Input: part model. Units: mm. Frame: model coordinates. A direction names the side the tool comes from. Coordinates: 2 decimals unless noted, no trailing zeros. Order: outer loops, then holes, each group sorted by start corner. A loop starts at its lowest first (then second) coordinate and runs counter-clockwise, first axis right, second up. Notation, with made-up numbers: M 57,-13 L 64,-13 A27 cw 64,8 Z; hole C 52.25,-15.5 d9. An arc over 180 degrees is marked long. Answer in a Markdown table with one row per item.
from build123d import *

# Parameters (mm, degrees)
F1_DEPTH = 9.271
F2_R     = 6.731
F3_DEPTH = 6.35


with BuildPart() as f1:
    # F0 (on Top) → F1 (new body)
    with BuildSketch(Plane.XY):
        with BuildLine():
            Line((16.51, 19.05), (-16.51, 19.05))
            ThreePointArc((-16.51, 19.05), (-18.306051, 18.306051), (-19.05, 16.51))
            Line((-19.05, 16.51), (-19.05, -16.51))
            ThreePointArc((-19.05, -16.51), (-18.306051, -18.306051), (-16.51, -19.05))
            Line((-16.51, -19.05), (16.51, -19.05))
            ThreePointArc((16.51, -19.05), (18.306051, -18.306051), (19.05, -16.51))
            Line((19.05, -16.51), (19.05, 16.51))
            ThreePointArc((19.05, 16.51), (18.306051, 18.306051), (16.51, 19.05))
        make_face()
    extrude(amount=F1_DEPTH)

    # F2 (on face) → F3 (cut)
    with BuildSketch(Plane.XY.offset(9.271)):
        Circle(F2_R)
    extrude(amount=-F3_DEPTH, mode=Mode.SUBTRACT)


solid = f1.part
1) Contact query for flat-ended pins moving along their axis: pin 1 (3 mm diameter, centred on x = -5, y = 15, fed in from -Z); pin 2 (6.5 mm diameter, centred on x = -1, y = 2, fed in from +Z). Output: stop coordinate, or through.
Resolved:
| item | result |
|---|---|
| pin 1 | stops at z = 0 |
| pin 2 | stops at z = 2.92 |
2) Material intervals for probe 1 along Y at (x, z) = (0, 8.75); probe 2 along X at (y, z) = (-0.5, 5.5); probe 3 along Z at (x, y) = (1, 2), sorted ascending.
Resolved:
| item | result |
|---|---|
| probe 1 | y = -19.05 to -6.73, 6.73 to 19.05 |
| probe 2 | x = -19.05 to -6.71, 6.71 to 19.05 |
| probe 3 | z = 0 to 2.92 |
3) Cut plane A-A, the plane z = 4.5. Output: boundary loops of the cut face in (x, y), and give its area (3 significant figures).
Resolved:
| item | result |
|---|---|
| outline | M -19.05,-16.51 A2.54 ccw -16.51,-19.05 L 16.51,-19.05 A2.54 ccw 19.05,-16.51 L 19.05,16.51 A2.54 ccw 16.51,19.05 L -16.51,19.05 A2.54 ccw -19.05,16.51 Z; hole C 0,0 d13.46 |
| area | 1,300 mm2 |
4) Reachability of faces 4 (the face through (0, 0, 2.921)), 5 (the face through (18.326, 18.286, 4.571)) from +Z, -Z, +X, -X, +Y, -Y: full face, straight path, thin tool, end or side. Return the list, or none.
Resolved:
| item | result |
|---|---|
| face 4 | +Z |
| face 5 | +Z, -Z, +X, +Y |
5) Cut plane B-B, the plane y = 0. Output: boundary loops of the cut face in (x, z), and give its area (3 significant figures).
Resolved:
| item | result |
|---|---|
| outline | M -19.05,0 L 19.05,0 L 19.05,9.27 L 6.73,9.27 L 6.73,2.92 L -6.73,2.92 L -6.73,9.27 L -19.05,9.27 Z |
| area | 268 mm2 |
6) Mould query, pull axis Y, two halves, no side actions, for faces 1 (the face through (0, 19.05, 5)), 2 (the face through (-5.34, -4.1, 6.14)), 3 (the face through (8, 0, 9.271)). Classes: +Y half, -Y half, draft (parallel to the pull), parting line (faces both ways), or undercut.
Resolved:
| item | result |
|---|---|
| face 1 | +Y half |
| face 2 | undercut |
| face 3 | draft |
